Autodesk Inventor part; units mm, degrees
ref_plane "YZ Plane" through (0, 0, 0) normal (1, 0, 0) x (0, 1, 0)
ref_plane "XZ Plane" through (0, 0, 0) normal (0, 1, 0) x (-1, 0, 0)
ref_plane "XY Plane" through (0, 0, 0) normal (0, 0, 1) x (1, 0, 0)
sketch "Sketch1" plane through (0, 0, 0) normal (0, 1, 0) x (-1, 0, 0)
  line L0 (38.1, 3.9053) -> (-38.1, 3.9052)
  line L1 (-38.1, 3.9052) -> (-38.1, -3.9053)
  line L2 (-38.1, -3.9053) -> (38.1, -3.9052)
  line L3 (38.1, -3.9052) -> (38.1, 3.9053)
  line L4 (38.1, 3.9053) -> (-38.1, -3.9053) construction
  line L5 (-38.1, 3.9052) -> (38.1, -3.9052) construction
  point P0 (0, 0)
  dimension "d0" = 76.2
  dimension "d1" = 7.8105
extrude "Extrusion1" add sketch "Sketch1" along normal blind 1.5875
sketch "Sketch2" plane through (0, 1.5875, 0) normal (0, 1, 0) x (1, 0, 0)
  line L0 (-38.1, -3.9053) -> (38.1, -3.9052)
  line L1 (-12.7, -3.9053) -> (-25.4, -3.9053)
  line L2 (-25.4, -3.9053) -> (-25.4, -2.3178)
  line L3 (-38.1, 3.9052) -> (-38.1, -3.9053)
  line L4 (-25.4, -2.3178) -> (-36.5125, -2.3178)
  line L5 (-36.5125, -2.3178) -> (-36.5125, 2.3177)
  line L6 (-36.5125, 2.3177) -> (36.5125, 2.3178)
  line L7 (36.5125, 2.3178) -> (36.5125, -2.3177)
  line L8 (36.5125, -2.3177) -> (22.225, -2.3177)
  line L9 (22.225, -2.3177) -> (22.225, -3.9052)
  line L10 (38.1, -3.9052) -> (38.1, 3.9053)
  line L11 (38.1, 3.9053) -> (-38.1, 3.9052)
  line L12 (-25.4, -3.9053) -> (-38.1, -3.9053)
  line L13 (-38.1, 3.9052) -> (38.1, 3.9053)
  line L14 (38.1, -3.9052) -> (22.225, -3.9052)
  line L15 (38.1, 3.9053) -> (38.1, -3.9052)
  line L16 (-38.1, -3.9053) -> (-38.1, 3.9052)
  point P0 (0, 0)
  dimension "d5" = 12.7
  dimension "d6" = 1.5875
  dimension "d7" = 1.5875
  dimension "d8" = 1.5875
  dimension "d9" = 1.5875
  dimension "d10" = 1.5875
extrude "Extrusion2" add sketch "Sketch2" along normal blind 68.2625 contours L3 L11 L10 L0 L9 L8 L7 L6 L5 L4 L2
sketch "Sketch3" plane through (38.1, 0, -3.9053) normal (0, 0, -1) x (-1, 0, 0)
  circle A0 centre (38.1, 52.3875) radius 2.4343
  circle A1 centre (38.1, 20.6375) radius 2.4343
  line L0 (0, 69.85) -> (76.2, 69.85)
  point P0 (38.1, 0)
  point P1 (38.1, 69.85)
  dimension "d13" = 31.75
  dimension "d14" = 17.4625
extrude "Extrusion3" cut sketch "Sketch3" against normal blind 68.2625
fillet "Fillet1" radius 3.175 2 edges at (38.1, 34.925, -3.9053) (-38.1, 34.925, -3.9052)
fillet "Fillet2" radius 3.175 2 edges at (-38.1, 34.925, 3.9053) (38.1, 34.925, 3.9052)
properties part number "Monitor Seat v1.0"
For this review, take the finished solid that the model builds, in its own axes (mm). A direction names the side the tool comes from. Coordinates: 2 decimals unless noted, no trailing zeros. Loops run counter-clockwise (first coordinate to the right, second up) from the corner with the lowest first, then second, coordinate; pieces in that order, holes last.
1. For faces 1 (the flat face through (-25.4, 35, 3)), 2 (the cylindrical face through (37.145, 34.436, -3)), 3 (the flat face through (-31, 35, 2.318)), list the 3-axis set-ups (+Z, -Z, +X, -X, +Y, -Y) from which the entire face can be reached by the end or side of a thin tool; tool diameter is ignored.
2. Add section A-A, the plane x = 0. Give the boundary of the cut face in (y, z).
3. Insertion check: P1, Ø6.5, axis at x = 0, y = 20.64, coming from the +Z side; P2, Ø2, axis at y = 12.5, z = -2.5, coming from the +X side; P3, Ø1.3, axis at y = 44.5, z = 3, coming from the +X side. Each pin has a flat end and moves straight along its axis. Give the tip position at first contact, or say it passes through.
4. Mouldability with a two-part tool opening along Z and no side actions: class faces 4 (the flat face through (29, 35, 2.318)), 5 (the cylindrical face through (37.145, 35.414, 3)), 6 (the cylindrical face through (-37.195, 34.436, -2.95)) as +Z half, -Z half, draft (parallel to the pull), parting line (faces both ways), or undercut.
5. Add section C-C, the plane x = 10.5. Give the boundary of the cut face in (y, z).
6. For line 1 (Y direction, x = 0, z = -2.7); line 2 (X direction, y = 56, z = -0.5); line 3 (Z direction, x = 25.5, y = 50.5), list the stretches that pass through material, from the lowest coordinate up.
Result:
1. face 1: +Z, +Y
1. face 2: -Z, +X, +Y, -Y
1. face 3: +Y
2. outline: (0, -3.91) - (18.2, -3.91) - (18.2, -2.32) - (1.59, -2.32) - (1.59, 3.91) - (0, 3.91) - close; (23.07, -3.91) - (49.95, -3.91) - (49.95, -2.32) - (23.07, -2.32) - close; (54.82, -3.91) - (69.85, -3.91) - (69.85, -2.32) - (54.82, -2.32) - close
3. P1: stops at z = -2.32
3. P2: stops at x = 38.01
3. P3: stops at x = 37.66
4. face 4: undercut
4. face 5: +Z half
4. face 6: -Z half
5. outline: (0, -3.91) - (69.85, -3.91) - (69.85, -2.32) - (1.59, -2.32) - (1.59, 3.91) - (0, 3.91) - close
6. line 1: y = 0 to 18.2, 23.07 to 49.95, 54.82 to 69.85
6. line 2: x = -38.1 to -36.51, 36.51 to 38.1
6. line 3: z = -3.91 to -2.32, 2.32 to 3.91
